Here's how the part is built. I have some questions about the finished solid (model axes, mm). A direction names the side the tool comes from. Give positions to 0.01 mm unless a question says otherwise; leave off trailing zeros. Write each loop counter-clockwise with the first axis right and the second up, starting at its lowest first coordinate (ties: lowest second). Pieces come first, ordered by that corner, then holes. Notation, with made-up numbers: (26.5, 70) - (32.5, 70) arc R20 cw to (32.5, 80) - close; hole circle Ø11 at (72.5, 59.25). An arc over 180 degrees is marked (long way). One line per item, written item: value. Start each with the question number.
1) We'd pull the mould along X, two halves only. Please class faces 4 (the cylindrical face through (-16.51, 3.46, 5)), 5 (the cylindrical face through (-10.605, -10.668, 4.092)), 6 (the cylindrical face through (-16.395, -16.332, 4.092)), 7 (the cylindrical face through (16.332, -16.395, 4.092)): +X half, -X half, draft (parallel to the pull), parting line (faces both ways), or undercut.
2) Imagine slicing it at C-C on y = -12. Write out the boundary of the cut face in (x, z).
3) Imagine slicing it at A-A on y = 3.35. Write out the boundary of the cut face in (x, z).
4) Imagine slicing it at B-B on x = 9. Write out the boundary of the cut face in (y, z), plus the area to 3 significant figures.
5) Please list where this line runs through material, in increasing order: L1, parallel to X at y = -6.5, z = 6.5. Write a range as [from, to].
6) Imagine slicing it at D-D on z = 3. Count the separate pieces of the cut face and the enclosed holes in it, plus the area to 3 significant figures.
7) On a 3-axis mill with a long thin cutter (end or side, diameter ignored), from which of +Z, -Z, +X, -X, +Y, -Y can I reach the whole of each face in a straight line? I mean faces 1 (the cylindrical face through (10.668, -10.605, 4.092)), 2 (the flat face through (-15.5, 4.2, 5.1)), 3 (the flat face through (-13.5, -4, 5)). Say none if no direction works.
8) I'm going to push a flat-ended pin straight in: P1, Ø1, axis at x = -13.5, y = 12.5, coming from the -Z side. Where does the tip first touch, or does it pass through?
from build123d import *

# Parameters (mm, degrees)
F0_W     = 2
F0_H     = 6.1
F0_H_2   = 2
F0_W_2   = 2.05
F0_H_3   = 5
F1_DEPTH = 8.3
F2_ANGLE = 180
F3_ANGLE = 180


with BuildPart() as f1:
    # F0 (on Top) → F1 (new body)
    with BuildSketch(Plane.XY):
        with BuildLine():
            ThreePointArc((-13.5, 9.45), (-14.5342970466, 9.5842970466), (-15.5, 9.9782816694))
            Line((-15.5, 9.9782816694), (-15.5, 9.45))
            Line((-15.5, 9.45), (-13.5, 9.45))
        make_face()
        with BuildLine():
            ThreePointArc((-9.45, 13.5), (-10.6362175362, 16.3637824638), (-13.5, 17.55))
            ThreePointArc((-13.5, 17.55), (-16.3637824638, 16.3637824638), (-17.55, 13.5))
            ThreePointArc((-17.55, 13.5), (-17.0001785669, 11.4625383439), (-15.5, 9.9782816694))
            Line((-15.5, 9.9782816694), (-15.5, 11.45))
            Line((-15.5, 11.45), (-13.5, 11.45))
            ThreePointArc((-13.5, 11.45), (-14.9495689014, 14.9495689014), (-11.45, 13.5))
            Line((-11.45, 13.5), (-9.45, 13.5))
        make_face()
        with BuildLine():
            Line((-15.5, 11.45), (-15.5, 9.9782816694))
            ThreePointArc((-15.5, 9.9782816694), (-14.5342970466, 9.5842970466), (-13.5, 9.45))
            Line((-13.5, 9.45), (-13.5, 11.45))
            Line((-13.5, 11.45), (-15.5, 11.45))
        make_face()
        with BuildLine():
            ThreePointArc((-15.5, 9.9782816694), (-17.0001785669, 11.4625383439), (-17.55, 13.5))
            Line((-17.55, 13.5), (-17.55, 8.35))
            Line((-17.55, 8.35), (-15.5, 8.35))
            Line((-15.5, 8.35), (-15.5, 9.45))
            Line((-15.5, 9.45), (-15.5, 9.9782816694))
        make_face()
        with Locations((-14.5, 0.3)):
            Rectangle(F0_W, F0_H)
        with Locations((-14.5, -3.75)):
            Rectangle(F0_W, F0_H_2)
        with BuildLine():
            ThreePointArc((-13.5, -9.45), (-16.3637824638, -10.6362175362), (-17.55, -13.5))
            ThreePointArc((-17.55, -13.5), (-16.3637824638, -16.3637824638), (-13.5, -17.55))
            ThreePointArc((-13.5, -17.55), (-10.6362175362, -16.3637824638), (-9.45, -13.5))
            Line((-9.45, -13.5), (-11.45, -13.5))
            ThreePointArc((-11.45, -13.5), (-14.9495689014, -14.9495689014), (-13.5, -11.45))
            Line((-13.5, -11.45), (-13.5, -9.45))
        make_face()
        with BuildLine():
            Line((-13.5, -17.55), (13.5, -17.55))
            ThreePointArc((13.5, -17.55), (10.6362175362, -16.3637824638), (9.45, -13.5))
            Line((9.45, -13.5), (-9.45, -13.5))
            ThreePointArc((-9.45, -13.5), (-10.6362175362, -16.3637824638), (-13.5, -17.55))
        make_face()
        with BuildLine():
            ThreePointArc((-9.45, -13.5), (-10.6362175362, -10.6362175362), (-13.5, -9.45))
            Line((-13.5, -9.45), (-13.5, -11.45))
            ThreePointArc((-13.5, -11.45), (-12.0504310986, -12.0504310986), (-11.45, -13.5))
            Line((-11.45, -13.5), (-9.45, -13.5))
        make_face()
        with BuildLine():
            ThreePointArc((13.5, -17.55), (16.3637824638, -16.3637824638), (17.55, -13.5))
            ThreePointArc((17.55, -13.5), (16.3637824638, -10.6362175362), (13.5, -9.45))
            Line((13.5, -9.45), (13.5, -11.45))
            ThreePointArc((13.5, -11.45), (14.9495689014, -12.0504310986), (15.55, -13.5))
            ThreePointArc((15.55, -13.5), (13.5, -15.55), (11.45, -13.5))
            Line((11.45, -13.5), (9.45, -13.5))
            ThreePointArc((9.45, -13.5), (10.6362175362, -16.3637824638), (13.5, -17.55))
        make_face()
        with BuildLine():
            Line((13.5, -11.45), (13.5, -9.45))
            ThreePointArc((13.5, -9.45), (10.6362175362, -10.6362175362), (9.45, -13.5))
            Line((9.45, -13.5), (11.45, -13.5))
            ThreePointArc((11.45, -13.5), (12.0504310986, -12.0504310986), (13.5, -11.45))
        make_face()
        with BuildLine():
            Line((17.55, 8.35), (17.55, 13.5))
            ThreePointArc((17.55, 13.5), (17.0001785669, 11.4625383439), (15.5, 9.9782816694))
            Line((15.5, 9.9782816694), (15.5, 9.45))
            Line((15.5, 9.45), (15.5, 8.35))
            Line((15.5, 8.35), (17.55, 8.35))
        make_face()
        with Locations((14.5, -3.75)):
            Rectangle(F0_W, F0_H_2)
        with Locations((14.5, 0.3)):
            Rectangle(F0_W, F0_H)
        with BuildLine():
            Line((15.5, 9.45), (15.5, 9.9782816694))
            ThreePointArc((15.5, 9.9782816694), (14.5342970466, 9.5842970466), (13.5, 9.45))
            Line((13.5, 9.45), (15.5, 9.45))
        make_face()
        with BuildLine():
            ThreePointArc((13.5, 9.45), (14.5342970466, 9.5842970466), (15.5, 9.9782816694))
            Line((15.5, 9.9782816694), (15.5, 11.45))
            Line((15.5, 11.45), (13.5, 11.45))
            Line((13.5, 11.45), (13.5, 9.45))
        make_face()
        with BuildLine():
            ThreePointArc((11.5, 9.9782816694), (12.4657029534, 9.5842970466), (13.5, 9.45))
            Line((13.5, 9.45), (13.5, 11.45))
            Line((13.5, 11.45), (11.5, 11.45))
            Line((11.5, 11.45), (11.5, 9.9782816694))
        make_face()
        with BuildLine():
            Line((11.5, 11.45), (10.0071501607, 11.45))
            ThreePointArc((10.0071501607, 11.45), (10.6567028733, 10.6158776986), (11.5, 9.9782816694))
            Line((11.5, 9.9782816694), (11.5, 11.45))
        make_face()
        with BuildLine():
            Line((11.45, 13.5), (9.45, 13.5))
            ThreePointArc((9.45, 13.5), (9.5917688241, 12.4378187182), (10.0071501607, 11.45))
            Line((10.0071501607, 11.45), (11.5, 11.45))
            Line((11.5, 11.45), (13.5, 11.45))
            ThreePointArc((13.5, 11.45), (12.0504310986, 12.0504310986), (11.45, 13.5))
        make_face()
        with BuildLine():
            ThreePointArc((17.55, 13.5), (16.3637824638, 16.3637824638), (13.5, 17.55))
            ThreePointArc((13.5, 17.55), (10.6362175362, 16.3637824638), (9.45, 13.5))
            Line((9.45, 13.5), (11.45, 13.5))
            ThreePointArc((11.45, 13.5), (13.5, 15.55), (15.55, 13.5))
            ThreePointArc((15.55, 13.5), (14.9495689014, 12.0504310986), (13.5, 11.45))
            Line((13.5, 11.45), (15.5, 11.45))
            Line((15.5, 11.45), (15.5, 9.9782816694))
            ThreePointArc((15.5, 9.9782816694), (17.0001785669, 11.4625383439), (17.55, 13.5))
        make_face()
        with BuildLine():
            ThreePointArc((9.45, 13.5), (10.6362175362, 16.3637824638), (13.5, 17.55))
            Line((13.5, 17.55), (-13.5, 17.55))
            ThreePointArc((-13.5, 17.55), (-10.6362175362, 16.3637824638), (-9.45, 13.5))
            Line((-9.45, 13.5), (9.45, 13.5))
        make_face()
        with BuildLine():
            ThreePointArc((-10.0071501607, 11.45), (-9.5917688241, 12.4378187182), (-9.45, 13.5))
            Line((-9.45, 13.5), (-11.45, 13.5))
            ThreePointArc((-11.45, 13.5), (-12.0504310986, 12.0504310986), (-13.5, 11.45))
            Line((-13.5, 11.45), (-11.5, 11.45))
            Line((-11.5, 11.45), (-10.0071501607, 11.45))
        make_face()
        with BuildLine():
            Line((-11.5, 11.45), (-13.5, 11.45))
            Line((-13.5, 11.45), (-13.5, 9.45))
            ThreePointArc((-13.5, 9.45), (-12.4657029534, 9.5842970466), (-11.5, 9.9782816694))
            Line((-11.5, 9.9782816694), (-11.5, 11.45))
        make_face()
        with BuildLine():
            ThreePointArc((-11.5, 9.9782816694), (-10.6567028733, 10.6158776986), (-10.0071501607, 11.45))
            Line((-10.0071501607, 11.45), (-11.5, 11.45))
            Line((-11.5, 11.45), (-11.5, 9.9782816694))
        make_face()
        with BuildLine():
            Line((-15.5, 3.35), (-17.55, 3.35))
            Line((-17.55, 3.35), (-17.55, -13.5))
            ThreePointArc((-17.55, -13.5), (-16.3637824638, -10.6362175362), (-13.5, -9.45))
            Line((-13.5, -9.45), (-13.5, -4.75))
            Line((-13.5, -4.75), (-15.5, -4.75))
            Line((-15.5, -4.75), (-15.5, -2.75))
            Line((-15.5, -2.75), (-15.5, 3.35))
        make_face()
        with Locations((-16.525, 5.85)):
            Rectangle(F0_W_2, F0_H_3)
        Polygon((-15.5, 9.45), (-15.5, 8.35), (-15.5, 3.35), (-13.5, 3.35), (-13.5, 9.45), align=None)
        with Locations((16.525, 5.85)):
            Rectangle(F0_W_2, F0_H_3)
        Polygon((15.5, 3.35), (15.5, 8.35), (15.5, 9.45), (13.5, 9.45), (13.5, 3.35), align=None)
        with BuildLine():
            Line((17.55, -13.5), (17.55, 3.35))
            Line((17.55, 3.35), (15.5, 3.35))
            Line((15.5, 3.35), (15.5, -2.75))
            Line((15.5, -2.75), (15.5, -4.75))
            Line((15.5, -4.75), (13.5, -4.75))
            Line((13.5, -4.75), (13.5, -9.45))
            ThreePointArc((13.5, -9.45), (16.3637824638, -10.6362175362), (17.55, -13.5))
        make_face()
    extrude(amount=F1_DEPTH)

    # F0 (on Top) → F2 (revolve)
    with BuildSketch(Plane.XY):
        with Locations((-16.525, 5.85)):
            Rectangle(F0_W_2, F0_H_3)
        Polygon((-15.5, 9.45), (-15.5, 8.35), (-15.5, 3.35), (-13.5, 3.35), (-13.5, 9.45), align=None)
        with Locations((-12.5, 6.4)):
            Rectangle(F0_W, F0_H)
        with BuildLine():
            Line((-11.5, 11.45), (-13.5, 11.45))
            Line((-13.5, 11.45), (-13.5, 9.45))
            ThreePointArc((-13.5, 9.45), (-12.4657029534, 9.5842970466), (-11.5, 9.9782816694))
            Line((-11.5, 9.9782816694), (-11.5, 11.45))
        make_face()
        with BuildLine():
            Line((-15.5, 11.45), (-15.5, 9.9782816694))
            ThreePointArc((-15.5, 9.9782816694), (-14.5342970466, 9.5842970466), (-13.5, 9.45))
            Line((-13.5, 9.45), (-13.5, 11.45))
            Line((-13.5, 11.45), (-15.5, 11.45))
        make_face()
        with BuildLine():
            ThreePointArc((11.5, 9.9782816694), (12.4657029534, 9.5842970466), (13.5, 9.45))
            Line((13.5, 9.45), (13.5, 11.45))
            Line((13.5, 11.45), (11.5, 11.45))
            Line((11.5, 11.45), (11.5, 9.9782816694))
        make_face()
        with Locations((12.5, 6.4)):
            Rectangle(F0_W, F0_H)
        with BuildLine():
            ThreePointArc((13.5, 9.45), (14.5342970466, 9.5842970466), (15.5, 9.9782816694))
            Line((15.5, 9.9782816694), (15.5, 11.45))
            Line((15.5, 11.45), (13.5, 11.45))
            Line((13.5, 11.45), (13.5, 9.45))
        make_face()
        with BuildLine():
            Line((-11.5, 9.45), (-11.5, 9.9782816694))
            ThreePointArc((-11.5, 9.9782816694), (-12.4657029534, 9.5842970466), (-13.5, 9.45))
            Line((-13.5, 9.45), (-11.5, 9.45))
        make_face()
        with BuildLine():
            ThreePointArc((-13.5, 9.45), (-14.5342970466, 9.5842970466), (-15.5, 9.9782816694))
            Line((-15.5, 9.9782816694), (-15.5, 9.45))
            Line((-15.5, 9.45), (-13.5, 9.45))
        make_face()
        with BuildLine():
            Line((15.5, 9.45), (15.5, 9.9782816694))
            ThreePointArc((15.5, 9.9782816694), (14.5342970466, 9.5842970466), (13.5, 9.45))
            Line((13.5, 9.45), (15.5, 9.45))
        make_face()
        with BuildLine():
            Line((11.5, 9.45), (13.5, 9.45))
            ThreePointArc((13.5, 9.45), (12.4657029534, 9.5842970466), (11.5, 9.9782816694))
            Line((11.5, 9.9782816694), (11.5, 9.45))
        make_face()
        with Locations((16.525, 5.85)):
            Rectangle(F0_W_2, F0_H_3)
        Polygon((15.5, 3.35), (15.5, 8.35), (15.5, 9.45), (13.5, 9.45), (13.5, 3.35), align=None)
    revolve(axis=Axis((0, 3.35, 0), (1, 0, 0)), revolution_arc=F2_ANGLE)

    # F0 (on Top) → F3 (revolve, cut)
    with BuildSketch(Plane.XY):
        Polygon((15.5, 3.35), (15.5, 8.35), (15.5, 9.45), (13.5, 9.45), (13.5, 3.35), align=None)
        with Locations((16.525, 5.85)):
            Rectangle(F0_W_2, F0_H_3)
        with Locations((12.5, 6.4)):
            Rectangle(F0_W, F0_H)
        with Locations((-12.5, 6.4)):
            Rectangle(F0_W, F0_H)
        Polygon((-15.5, 9.45), (-15.5, 8.35), (-15.5, 3.35), (-13.5, 3.35), (-13.5, 9.45), align=None)
        with Locations((-16.525, 5.85)):
            Rectangle(F0_W_2, F0_H_3)
    revolve(axis=Axis((0, 3.35, 0), (1, 0, 0)), revolution_arc=F3_ANGLE, mode=Mode.SUBTRACT)


solid = f1.part
Numbers:
1. face 4: draft
1. face 5: undercut
1. face 6: -X half
1. face 7: +X half
2. outline: (-17.55, 0) - (-14.9, 0) - (-14.9, 8.3) - (-17.55, 8.3) - close; (-12.1, 0) - (-9.74, 0) - (-9.74, 8.3) - (-12.1, 8.3) - close; (9.74, 0) - (12.1, 0) - (12.1, 8.3) - (9.74, 8.3) - close; (14.9, 0) - (17.55, 0) - (17.55, 8.3) - (14.9, 8.3) - close
3. outline: (-17.55, 5) - (-15.5, 5) - (-15.5, 6.1) - (-11.5, 6.1) - (-11.5, 8.1) - (-13.5, 8.1) - (-13.5, 8.3) - (-17.55, 8.3) - close; (11.5, 6.1) - (15.5, 6.1) - (15.5, 5) - (17.55, 5) - (17.55, 8.3) - (13.5, 8.3) - (13.5, 8.1) - (11.5, 8.1) - close
4. outline: (-17.55, 0) - (-13.5, 0) - (-13.5, 8.3) - (-17.55, 8.3) - close; (13.5, 0) - (17.55, 0) - (17.55, 8.3) - (13.5, 8.3) - close
4. area: 67.2 mm^2
5. L1: [-17.55, -13.5], [13.5, 17.55]
6. separate pieces: 2
6. enclosed holes: 4
6. area: 425 mm^2
7. face 1: +Z, -Z
7. face 2: -Z
7. face 3: +Z
8. P1: through
